from build123d import *

# Parameters (mm, degrees)
SKETCH2_R           = 2.65
BOSS_EXTRUDE1_DEPTH = 2
BOSS_EXTRUDE2_DEPTH = 2
CHAMFER1_SIZE       = 4.5
CHAMFER1_SIZE2      = 0.956504528
BOSS_EXTRUDE3_START = 1
BOSS_EXTRUDE3_DEPTH = 1
SKETCH21_W          = 20.8
SKETCH21_H          = 20.8
BOSS_EXTRUDE4_DEPTH = 10


with BuildPart() as part:
    # Sketch2 → Boss-Extrude1 (new body)
    with BuildSketch(Plane(origin=(0, 0, 0), x_dir=(1, 0, 0), z_dir=(0, 1, 0))):
        with BuildLine():
            Line((-15.984695958, -228.591802117), (-17.334483725, -247.89466649))
            ThreePointArc((-17.334483725, -247.89466649), (0, -248.5), (17.334483725, -247.89466649))
            Line((17.334483725, -247.89466649), (15.984695958, -228.591802117))
            ThreePointArc((15.984695958, -228.591802117), (0, -229.15), (-15.984695958, -228.591802117))
        make_face()
        with Locations(Location((0, -236.25, 0), (0, 0, 270))):
            Circle(SKETCH2_R, mode=Mode.SUBTRACT)
    extrude(amount=BOSS_EXTRUDE1_DEPTH)

    # Sketch3 → Boss-Extrude2 (add)
    with BuildSketch(Plane(origin=(0, 0, 0), x_dir=(1, 0, 0), z_dir=(0, 1, 0))):
        with BuildLine():
            Line((-15.705670063, -224.601545916), (-15.984695958, -228.591802117))
            ThreePointArc((-15.984695958, -228.591802117), (0, -229.15), (15.984695958, -228.591802117))
            Line((15.984695958, -228.591802117), (15.705670063, -224.601545916))
            ThreePointArc((15.705670063, -224.601545916), (0, -225.15), (-15.705670063, -224.601545916))
        make_face()
    extrude(amount=BOSS_EXTRUDE2_DEPTH)

    # Chamfer1
    chamfer1_edges = [part.edges().sort_by_distance(p)[0] for p in [
        (0, 0, 225.15),
    ]]
    chamfer1_side = [part.faces().sort_by_distance(p)[0] for p in [
        (16.100023839, 0, 236.277479174),
    ]]
    chamfer(chamfer1_edges, length=CHAMFER1_SIZE, length2=CHAMFER1_SIZE2, reference=chamfer1_side[0])

    # Sketch4 → Boss-Extrude3 (add)
    with BuildSketch(Plane.XZ.offset(BOSS_EXTRUDE3_START)):
        with BuildLine():
            Line((-17.334483725, 247.89466649), (-17.038018712, 243.655019276))
            ThreePointArc((-17.038018712, 243.655019276), (0, 244.25), (17.038018712, 243.655019276))
            Line((17.038018712, 243.655019276), (17.334483725, 247.89466649))
            ThreePointArc((17.334483725, 247.89466649), (0, 248.5), (-17.334483725, 247.89466649))
        make_face()
    extrude(amount=-BOSS_EXTRUDE3_DEPTH)

    # Sketch20 → CSK for M3.5 Flat Head Machine Screw2 (revolve, cut)
    with BuildSketch(Plane(origin=(0, 2, 236.25), x_dir=(0, 0, 1), z_dir=(1, 0, 0))):
        Polygon((0, 0), (0, 3), (1.85, 3), (1.85, 2.25), (4.1, 0), align=None)
    revolve(axis=Axis((0, 8.35, 236.25), (0, -1, 0)), mode=Mode.SUBTRACT)

    # Sketch21 → Boss-Extrude4 (add)
    with BuildSketch(Plane(origin=(0, 2, 0), x_dir=(1, 0, 0), z_dir=(0, 1, 0))):
        with BuildLine():
            Line((17.334483725, -247.89466649), (15.705670063, -224.601545916))
            ThreePointArc((15.705670063, -224.601545916), (0, -225.15), (-15.705670063, -224.601545916))
            Line((-15.705670063, -224.601545916), (-17.334483725, -247.89466649))
            ThreePointArc((-17.334483725, -247.89466649), (0, -248.5), (17.334483725, -247.89466649))
        make_face()
        with Locations((0, -236.25)):
            Rectangle(SKETCH21_W, SKETCH21_H, mode=Mode.SUBTRACT)
    extrude(amount=BOSS_EXTRUDE4_DEPTH)


solid = part.part
Model file for the job. Use its own axes, mm. A direction names the side the tool comes from. Give positions to 0.01 mm unless a question says otherwise; leave off trailing zeros. Loops run counter-clockwise (first coordinate to the right, second up) from the corner with the lowest first, then second, coordinate; pieces in that order, holes last. Notation, with made-up numbers: (27, 17.25) -> (45, 17.25) arc R17 ccw to (45, 25.25) -> close; hole circle Ø7 at (-9.5, -27.75). An arc over 180 degrees is marked (long way). Use a Markdown table: item, result. Add a question column.
(1) Slice it at C-C on y = 6.75. List the corners of the cut face in (x, z).
(2) Mould opens along X. For faces 4 (the flat face through (0, 12, 247)), 5 (the flat face through (-10.4, 7, 236)), 6 (the cylindrical face through (-0.2, 5.4, 248.5)), 7 (the cylindrical face through (0.22, 6.4, 225.15)) say: +X half, -X half, draft (parallel to the pull), parting line (faces both ways), or undercut.
(3) Slice it at B-B on z = 236.25. List the corners of the cut face in (x, y).
(4) Tool access for faces 1 (the cylindrical face through (-0.24, -0.51, 244.25)), 2 (the flat face through (0, -1, 246)), 3 (the flat face through (10.4, 7, 236)): list every direction of +Z, -Z, +X, -X, +Y, -Y with a clear straight run to the whole face (end or side of a thin tool).
(5) Wall check: line 1 along Z through (x, y) = (0.5, 5.5); line 2 along Y through (x, z) = (-12, 232.25); line 3 along Y through (x, z) = (-1, 243.25). Give the ranges that are in metal, low to high.
(6) Slice it at A-A on x = 0. List the corners of the cut face in (y, z).
(7) Drop flat-ended pins along their axis: pin 1 Ø12 at (x, z) = (-1, 233) entering from +Y; pin 2 Ø4 at (y, z) = (1.5, 238) entering from -X; pin 3 Ø3 at (y, z) = (7, 232) entering from -X. Give the stop position or say it passes through.
Filled sheet:
| question | item | result |
|---|---|---|
| 1 | outline | (-17.33, 247.89) -> (-15.71, 224.6) arc R225.15 cw to (15.71, 224.6) -> (17.33, 247.89) arc R248.5 ccw to start; hole (-10.4, 225.85) -> (10.4, 225.85) -> (10.4, 246.65) -> (-10.4, 246.65) -> close |
| 2 | face 4 | draft |
| 2 | face 5 | undercut |
| 2 | face 6 | parting line |
| 2 | face 7 | undercut |
| 3 | outline | (-16.52, 0) -> (-2.65, 0) -> (-2.65, 0.55) -> (-4.1, 2) -> (-10.4, 2) -> (-10.4, 12) -> (-16.52, 12) -> close; (2.65, 0) -> (16.52, 0) -> (16.52, 12) -> (10.4, 12) -> (10.4, 2) -> (4.1, 2) -> (2.65, 0.55) -> close |
| 4 | face 1 | -Z, -Y |
| 4 | face 2 | +Z, -Z, +X, -X, -Y |
| 4 | face 3 | +Y |
| 5 | line 1 | 225.15 to 225.85, 246.65 to 248.5 |
| 5 | line 2 | 0 to 12 |
| 5 | line 3 | 0 to 2 |
| 6 | outline | (-1, 244.25) -> (0, 244.25) -> (0, 238.9) -> (0.55, 238.9) -> (2, 240.35) -> (2, 246.65) -> (12, 246.65) -> (12, 248.5) -> (-1, 248.5) -> close; (0, 229.65) -> (0.96, 225.15) -> (12, 225.15) -> (12, 225.85) -> (2, 225.85) -> (2, 232.15) -> (0.55, 233.6) -> (0, 233.6) -> close |
| 7 | pin 1 | y = 2 |
| 7 | pin 2 | x = -16.78 |
| 7 | pin 3 | x = -16.33 |
